Check sheet for the drawn part. Datum: minimum x, y, z corner. Units: mm. A direction names the side the tool comes from. Give positions to 0.01 mm unless a question says otherwise; leave off trailing zeros. Order: outer loops, then holes, each group sorted by start corner. A loop starts at its lowest first (then second) coordinate and runs counter-clockwise, first axis right, second up. Notation, with made-up numbers: (44, -31.75) -> (61, -31.75) arc R9 cw to (61, -27.75) -> close; hole circle Ø3 at (-3.75, 15.25). An arc over 180 degrees is marked (long way). Answer in a Markdown table with one row per item. Add a question column.
(1) Set-up check for the marked faces 1, 2, 3 and 4: record each of +Z, -Z, +X, -X, +Y, -Y from which the full face is reachable in a straight line by a thin tool's end or side.
(2) Thickness scan on L1, parallel to Y at x = 12.5, z = 1.8; L2, parallel to Y at x = 25.5, z = 2.45; L3, parallel to X at y = 9.5, z = 1.7. Record the ranges inside material, lowest first. Write a range as [from, to].
(3) Cross-section at A-A (y = 15). Record the cut outline in (x, z), then the cut area to 3 significant figures.
(4) Cross-section at D-D (z = 2.5). State how many separate pieces and enclosed holes the cut face has, then the cut area to 3 significant figures.
(5) Go/stop test with flat-tipped pins: pin 1 (1.5 mm diameter, centred on x = 24, z = 3.5, fed in from +Y); pin 2 (2.5 mm diameter, centred on x = 24.5, z = 2.5, fed in from -Y). Record where each tip stops, or that it passes through.
(6) Cross-section at C-C (x = 28.5). Record the cut outline in (y, z), then the cut area to 3 significant figures.
(7) Cross-section at B-B (x = 17). Record the cut outline in (y, z).
(8) Release check for a two-part mould opening along X. For the marked faces 5, 6, 7 and 8 record: released by +X, released by -X, zero draft, split by the parting line, or undercut.
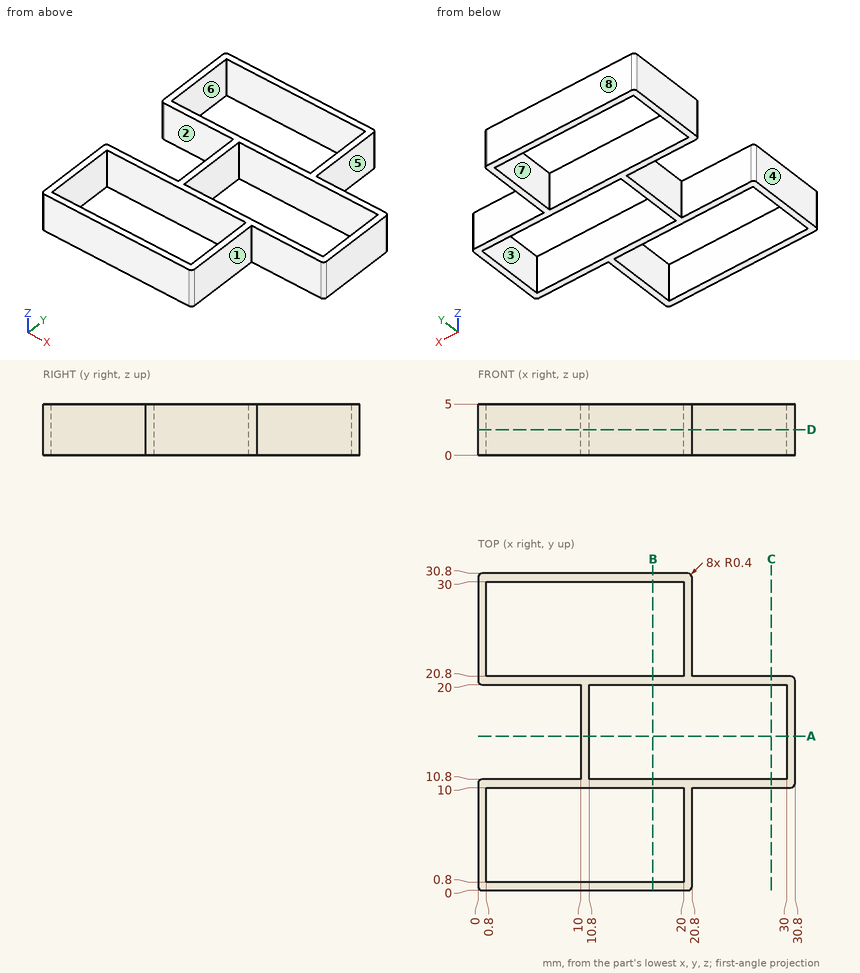
Answer below:
| question | item | result |
|---|---|---|
| 1 | face 1 | +Z, -Z, +X, -Y |
| 1 | face 2 | +Z, -Z, -X |
| 1 | face 3 | +Z, -Z |
| 1 | face 4 | +Z, -Z, -X, +Y, -Y |
| 2 | L1 | y = [0, 0.8], [10, 10.8], [20, 20.8], [30, 30.8] |
| 2 | L2 | y = [10, 10.8], [20, 20.8] |
| 2 | L3 | x = [0, 0.8], [20, 20.8] |
| 3 | outline | (10, 0) -> (10.8, 0) -> (10.8, 5) -> (10, 5) -> close; (30, 0) -> (30.8, 0) -> (30.8, 5) -> (30, 5) -> close |
| 3 | area | 8.00 mm² |
| 4 | separate pieces | 1 |
| 4 | enclosed holes | 3 |
| 4 | area | 126 mm² |
| 5 | pin 1 | stops at y = 20.8 |
| 5 | pin 2 | stops at y = 10 |
| 6 | outline | (10, 0) -> (10.8, 0) -> (10.8, 5) -> (10, 5) -> close; (20, 0) -> (20.8, 0) -> (20.8, 5) -> (20, 5) -> close |
| 6 | area | 8.00 mm² |
| 7 | outline | (0, 0) -> (0.8, 0) -> (0.8, 5) -> (0, 5) -> close; (10, 0) -> (10.8, 0) -> (10.8, 5) -> (10, 5) -> close; (20, 0) -> (20.8, 0) -> (20.8, 5) -> (20, 5) -> close; (30, 0) -> (30.8, 0) -> (30.8, 5) -> (30, 5) -> close |
| 8 | face 5 | released by +X |
| 8 | face 6 | undercut |
| 8 | face 7 | undercut |
| 8 | face 8 | zero draft |
